The model under review builds one solid part; all positions refer to its coordinate system, in mm. A direction names the side the tool comes from. Round coordinates to 2 decimals unless told otherwise and drop trailing zeros. Write each loop counter-clockwise with the first axis right and the second up, starting at its lowest first coordinate (ties: lowest second). Pieces come first, ordered by that corner, then holes. Notation, with made-up numbers: (-10.75, -16.5) - (4.25, -16.5) arc R20 ccw to (4.25, -7.5) - close; hole circle Ø1 at (69, -8). An arc over 180 degrees is marked (long way). Write each question's results on one line, items separated by ' | '.
```python
from build123d import *

# Parameters (mm, degrees)
SKETCH1_R           = 5
BOSS_EXTRUDE1_DEPTH = 4.5
CUT_EXTRUDE2_REACH  = 60.696
SKETCH3_R           = 1.6
SKETCH1_4_R         = 20
SKETCH1_4_R_2       = 5
BOSS_EXTRUDE2_DEPTH = 10.5
BOSS_EXTRUDE3_START = 10.5
SKETCH4_R           = 23
SKETCH4_R_2         = 5
BOSS_EXTRUDE3_DEPTH = 1
SKETCH2_R           = 13
CUT_EXTRUDE1_DEPTH  = 4


with BuildPart() as part:
    # Sketch1 → Boss-Extrude1 (new body)
    with BuildSketch(Plane(origin=(0, 0, 0), x_dir=(1, 0, 0), z_dir=(0, 1, 0))):
        with BuildLine():
            Line((-4.841786735, 51.247838615), (-11.080979808, 27.038904937))
            ThreePointArc((-11.080979808, 27.038904937), (-13.986571903, 17.837473452), (-17.860571099, 9))
            ThreePointArc((-17.860571099, 9), (0, -20), (17.860571099, 9))
            ThreePointArc((17.860571099, 9), (13.986571903, 17.837473452), (11.080979808, 27.038904937))
            Line((11.080979808, 27.038904937), (4.841786735, 51.247838615))
            ThreePointArc((4.841786735, 51.247838615), (0, 55), (-4.841786735, 51.247838615))
        make_face()
        with Locations(Location((0, 0, 0), (0, 0, 270))):
            Circle(SKETCH1_R, mode=Mode.SUBTRACT)
    extrude(amount=BOSS_EXTRUDE1_DEPTH)

    # Sketch3 → Cut-Extrude2 (cut, up to next)
    with BuildSketch(Plane(origin=(0, 0, 0), x_dir=(1, 0, 0), z_dir=(0, 1, 0)), mode=Mode.PRIVATE) as cut_extrude2_sk1:
        with Locations(Location((0, 50.305422276, 0), (0, 0, 270))):
            Circle(SKETCH3_R)
    cut_extrude2_tool1 = extrude(cut_extrude2_sk1.sketch, amount=CUT_EXTRUDE2_REACH, mode=Mode.PRIVATE) & part.part
    add(cut_extrude2_tool1.solids().sort_by_distance((0, 0, -50.305422))[0], mode=Mode.SUBTRACT)

    # Sketch1<4> → Boss-Extrude2 (add)
    with BuildSketch(Plane(origin=(0, 0, 0), x_dir=(1, 0, 0), z_dir=(0, 1, 0))):
        with Locations(Location((0, 0, 0), (0, 0, 26.74368395))):
            Circle(SKETCH1_4_R)
        with Locations(Location((0, 0, 0), (0, 0, 270))):
            Circle(SKETCH1_4_R_2, mode=Mode.SUBTRACT)
    extrude(amount=BOSS_EXTRUDE2_DEPTH)

    # Sketch4 → Boss-Extrude3 (add)
    with BuildSketch(Plane(origin=(0, 0, 0), x_dir=(1, 0, 0), z_dir=(0, 1, 0)).offset(BOSS_EXTRUDE3_START)):
        with Locations(Location((0, 0, 0), (0, 0, 270))):
            Circle(SKETCH4_R)
        with Locations(Location((0, 0, 0), (0, 0, 270))):
            Circle(SKETCH4_R_2, mode=Mode.SUBTRACT)
    extrude(amount=BOSS_EXTRUDE3_DEPTH)

    # Sketch2 → Cut-Extrude1 (cut)
    with BuildSketch(Plane(origin=(0, 0, 0), x_dir=(1, 0, 0), z_dir=(0, 1, 0))):
        with Locations(Location((0, 0, 0), (0, 0, 270))):
            Circle(SKETCH2_R)
    extrude(amount=CUT_EXTRUDE1_DEPTH, mode=Mode.SUBTRACT)


solid = part.part
```
Q1. Insertion check: P1, Ø4, axis at y = 10, z = 1, coming from the +X side; P2, Ø1, axis at x = 14, y = 2, coming from the +Z side; P3, Ø2, axis at x = -3, y = 7.5, coming from the -Z side; P4, Ø4, axis at x = 8.5, z = -22.5, coming from the -Y side. Each pin has a flat end and moves straight along its axis. Give the tip position at first contact, or say it passes through.
Evaluation:
P1: stops at x = 23 | P2: stops at z = 14.76 | P3: stops at z = -19.9 | P4: stops at y = 0
Q2. We need section C-C (y = 6). State the section outline as (x, z) points.
Evaluation:
outline: circle Ø40 at (0, 0); hole circle Ø10 at (0, 0)
Q3. For probe 1 along Z at (x, y) = (0, 6.5); probe 2 along X at (y, z) = (2.9, 0), list the stretches that pass through material, from the lowest coordinate up.
Evaluation:
probe 1: z = -20 to -5, 5 to 20 | probe 2: x = -20 to -13, 13 to 20
Q4. We need section B-B (z = 0). State the section outline as (x, y) points, plus the area to 3 significant figures.
Evaluation:
outline: (-23, 10.5) - (-20, 10.5) - (-20, 0) - (-13, 0) - (-13, 4) - (-5, 4) - (-5, 11.5) - (-23, 11.5) - close; (5, 4) - (13, 4) - (13, 0) - (20, 0) - (20, 10.5) - (23, 10.5) - (23, 11.5) - (5, 11.5) - close | area: 287 mm^2
Q5. The part is to be moulded in two halves that separate along Z. For faces 1 (the cylindrical face through (0.07, 2.218, -51.904)), 2 (the cylindrical face through (4.914, 5.176, 19.387)), 3 (the cylindrical face through (-13.94, 2.22, -17.96)), say which applies: released by +Z, released by -Z, zero draft, split by the parting line, or undercut.
Evaluation:
face 1: undercut | face 2: split by the parting line | face 3: released by -Z
Q6. We need section D-D (x = 8.5). State the section outline as (y, z) points, plus the area to 3 significant figures.
Evaluation:
outline: (0, -37.05) - (4.5, -37.05) - (4.5, -18.1) - (10.5, -18.1) - (10.5, -21.37) - (11.5, -21.37) - (11.5, 21.37) - (10.5, 21.37) - (10.5, 18.1) - (0, 18.1) - (0, 9.84) - (4, 9.84) - (4, -9.84) - (0, -9.84) - close | area: 430 mm^2
Q7. Tool access review of faces 4 (the cylindrical face through (14.034, 2.218, -17.711)), 5 (the cylindrical face through (-7.91, 1.972, -10.316)), 6 (the flat face through (19, 10.5, -7)): name each direction out of +Z, -Z, +X, -X, +Y, -Y from which nothing blocks a thin tool from reaching the whole face with its end or side.
Evaluation:
face 4: -Z, +X, -Y | face 5: -Y | face 6: none
Q8. We need section A-A (x = 0). State the section outline as (y, z) points.
Evaluation:
outline: (0, -55) - (4.5, -55) - (4.5, -51.91) - (0, -51.91) - close; (0, -48.71) - (4.5, -48.71) - (4.5, -20) - (10.5, -20) - (10.5, -23) - (11.5, -23) - (11.5, -5) - (4, -5) - (4, -13) - (0, -13) - close; (0, 13) - (4, 13) - (4, 5) - (11.5, 5) - (11.5, 23) - (10.5, 23) - (10.5, 20) - (0, 20) - close
